The drawing under review shows one solid part. Ordinate dimensions are in mm from its lowest x, y, z. Give positions to 0.01 mm unless a question says otherwise; leave off trailing zeros. Write each loop counter-clockwise with the first axis right and the second up, starting at its lowest first coordinate (ties: lowest second). Pieces come first, ordered by that corner, then holes. Notation, with made-up numbers: (-31.5, -21) - (8.5, -21) arc R12 ccw to (8.5, -9) - close; hole circle Ø7 at (29, -31.5). An arc over 180 degrees is marked (long way). Write each question's results on one line, items separated by ' | '. Start each with the question number.
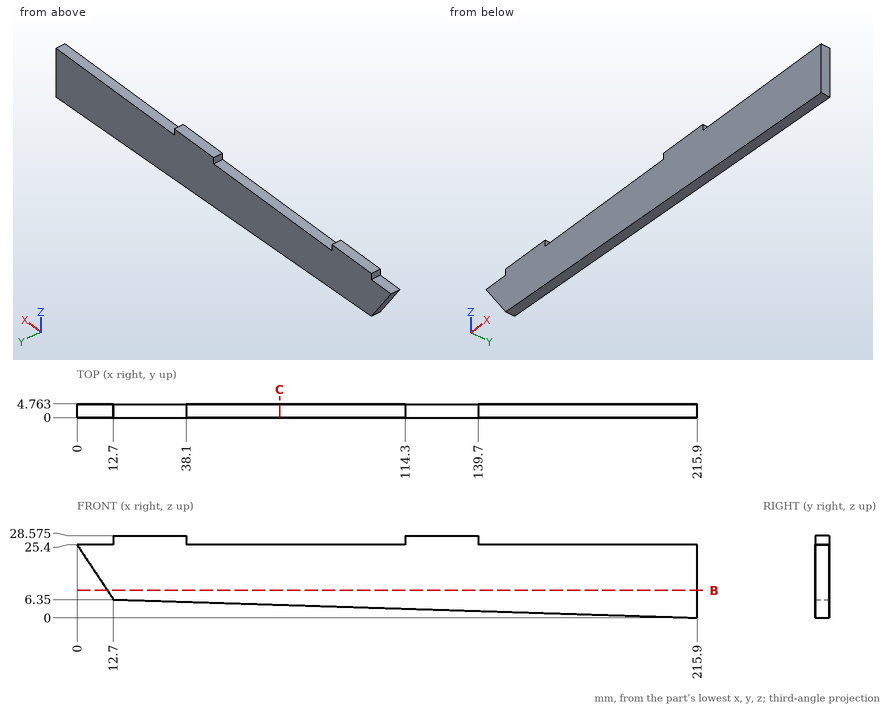
Q1. Add section C-C on x = 70.5. State the section outline as (y, z) points.
Q2. Add section B-B on z = 9.5. State the section outline as (x, y) points.
Q3. Insertion check: P1, Ø1.6, axis at y = 3, z = 27, coming from the +X side; P2, Ø1.6, axis at y = 2, z = 27.5, coming from the -X side; P3, Ø2.5, axis at x = 88, y = 2, coming from the +Z side. Each pin has a flat end and moves straight along its axis. Give the tip position at first contact, or say it passes through.
Q4. For line 1 along X through (y, z) = (3.8, 25.5); line 2 along Z through (x, y) = (81, 3.35) (1 decimal); line 3 along X through (y, z) = (0.6, 12.5), list the stretches that pass through material, from the lowest coordinate up. Write a range as [from, to].
Result:
1) outline: (0, 4.54) - (4.76, 4.54) - (4.76, 25.4) - (0, 25.4) - close
2) outline: (10.6, 0) - (215.9, 0) - (215.9, 4.76) - (10.6, 4.76) - close
3) P1: stops at x = 139.7 | P2: stops at x = 12.7 | P3: stops at z = 25.4
4) line 1: x = [12.7, 38.1], [114.3, 139.7] | line 2: z = [4.2, 25.4] | line 3: x = [8.6, 215.9]
